Can you work these out from the model? Positions are in its coordinate system, mm. Face numbers are marked on the shaded views. A direction names the side the tool comes from. Give positions to 0.01 mm unless a question says otherwise; leave off trailing zeros. Order: outer loops, then holes, each group sorted by start corner. A loop starts at its lowest first (then second) coordinate and runs counter-clockwise, first axis right, second up. Notation, with made-up numbers: (39.5, 80.25) - (46.5, 80.25) arc R15 cw to (46.5, 89.25) - close; hole circle Ø5 at (26.5, 21.25). An arc over 180 degrees is marked (long way). Return JSON: item names as keys, results as strings.
Autodesk Inventor part; units mm, degrees
ref_plane "YZ Plane" through (0, 0, 0) normal (1, 0, 0) x (0, 1, 0)
ref_plane "XZ Plane" through (0, 0, 0) normal (0, 1, 0) x (-1, 0, 0)
ref_plane "XY Plane" through (0, 0, 0) normal (0, 0, 1) x (1, 0, 0)
sketch "Sketch1" plane through (0, 0, 0) normal (0, 1, 0) x (-1, 0, 0)
  line L0 (6.35, -3.6662) -> (0, -7.3323)
  line L1 (0, -7.3323) -> (-6.35, -3.6662)
  line L2 (-6.35, -3.6662) -> (-6.35, 3.6662)
  line L3 (-6.35, 3.6662) -> (0, 7.3323)
  line L4 (0, 7.3323) -> (6.35, 3.6662)
  line L5 (6.35, 3.6662) -> (6.35, -3.6662)
  line L6 (-4.8895, 2.823) -> (0, 5.6459)
  line L7 (0, 5.6459) -> (4.8895, 2.823)
  line L8 (4.8895, 2.823) -> (4.8895, -2.823)
  line L9 (4.8895, -2.823) -> (0, -5.6459)
  line L10 (0, -5.6459) -> (-4.8895, -2.823)
  line L11 (-4.8895, -2.823) -> (-4.8895, 2.823)
  point P0 (0, 0)
  point P1 (0, 0)
  point P2 (0, 0)
  dimension "d0" = 9.779
  dimension "d1" = 12.7
extrude "Extrusion1" add sketch "Sketch1" along normal blind 15.875
chamfer "Chamfer1" distance 0.4 angle 45 24 edges at (-3.175, 0, 5.4993) (3.175, 0, 5.4993) (6.35, 0, 0) (3.175, 0, -5.4993) (-3.175, 0, -5.4993) (-6.35, 0, 0) (-2.4447, 0, -4.2344) (2.4448, 0, -4.2344) (4.8895, 0, 0) (2.4447, 0, 4.2344) (-2.4447, 0, 4.2344) (-4.8895, 0, 0) (-4.8895, 15.875, 0) (-2.4447, 15.875, 4.2344) (2.4447, 15.875, 4.2344) (4.8895, 15.875, 0) (2.4448, 15.875, -4.2344) (-2.4447, 15.875, -4.2344) (-3.175, 15.875, -5.4993) (-6.35, 15.875, 0) (-3.175, 15.875, 5.4993) (3.175, 15.875, 5.4993) (6.35, 15.875, 0) (3.175, 15.875, -5.4993)
properties part number "0_5_Hex_0_375_Hex_Adapter" material "Aluminum 6061"
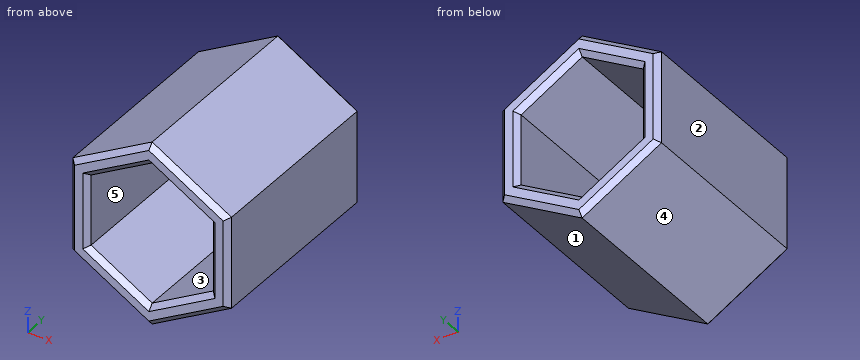
1. For pin 1 Ø2 at (x, y) = (-3, 2) entering from -Z; pin 2 Ø1.5 at (x, y) = (-4, 10) entering from -Z, each with a flat end and sliding along its axis, tell me the tip position at first contact or that it passes through.
Checks:
{"pin 1": "z = -6.18", "pin 2": "z = -5.46"}
2. Suppose I cut it at B-B (y = 3.75). List the corners of the cut face in (x, z) for me, plus the area to 3 significant figures.
Checks:
{"outline": "(-6.35, -3.67) - (0, -7.33) - (6.35, -3.67) - (6.35, 3.67) - (0, 7.33) - (-6.35, 3.67) - close; hole (-4.89, -2.82) - (0, -5.65) - (4.89, -2.82) - (4.89, 2.82) - (0, 5.65) - (-4.89, 2.82) - close", "area": "56.9 mm^2"}
3. Suppose I cut it at C-C (x = -2.5). List the corners of the cut face in (y, z) for me (3 decimals).
Checks:
{"outline": "(0, -5.427) - (0.4, -5.889) - (15.475, -5.889) - (15.875, -5.427) - (15.875, -4.664) - (15.475, -4.203) - (0.4, -4.203) - (0, -4.664) - close; (0, 4.664) - (0.4, 4.203) - (15.475, 4.203) - (15.875, 4.664) - (15.875, 5.427) - (15.475, 5.889) - (0.4, 5.889) - (0, 5.427) - close"}
4. On a 3-axis mill with a long thin cutter (end or side, diameter ignored), from which of +Z, -Z, +X, -X, +Y, -Y can I reach the whole of each face in a straight line? I mean the marked faces 4 and 5. Say none if no direction works.
Checks:
{"face 4": "-Z, -X, +Y, -Y", "face 5": "+Y, -Y"}
5. Suppose I cut it at D-D (z = -6.5). List the corners of the cut face in (x, y) for me (3 decimals), plus the area to 3 significant figures.
Checks:
{"outline": "(-1.442, 0.4) - (-0.642, 0) - (0.642, 0) - (1.442, 0.4) - (1.442, 15.475) - (0.642, 15.875) - (-0.642, 15.875) - (-1.442, 15.475) - close", "area": "45.1 mm^2"}
6. If I drill on L1, parallel to X at y = 12, z = -2.25; L2, parallel to Z at x = -1.5, y = 2; L3, parallel to X at y = 14.5, z = -3, over which ranges is the centre line in solid material (lowest first)? Write a range as [from, to].
Checks:
{"L1": "[-6.35, -4.89], [4.89, 6.35]", "L2": "[-6.47, -4.78], [4.78, 6.47]", "L3": "[-6.35, -4.58], [4.58, 6.35]"}
7. Thinking about a two-plate mould opening in Z: for the marked faces 1, 2 and 3, which applies, +Z half, -Z half, draft (parallel to the pull), parting line (faces both ways), or undercut?
Checks:
{"face 1": "-Z half", "face 2": "draft", "face 3": "undercut"}
